Design review of the part built by this model. Coordinates are the model's own, in mm. A direction names the side the tool comes from. Coordinates: 2 decimals unless noted, no trailing zeros. Write each loop counter-clockwise with the first axis right and the second up, starting at its lowest first coordinate (ties: lowest second). Pieces come first, ordered by that corner, then holes.
Q1. Take a section at D-D, the plane z = 0. Write out the cut boundary in (x, y).
Q2. For pin 1 Ø5 at (x, z) = (14.5, -1.5) entering from -Y; pin 2 Ø3 at (y, z) = (4.5, 2) entering from +X; pin 3 Ø3 at (y, z) = (3, 0.5) entering from -X; pin 4 Ø1.5 at (x, z) = (-14, -3.5) entering from -Y, all flat-tipped, find the tip position at first contact; note any pin that passes through.
Q3. For L1, parallel to X at y = 0.45, z = -3.5; L2, parallel to Y at x = 13, z = -5; L3, parallel to X at y = -8, z = -3.5, list the stretches that pass through material, from the lowest coordinate up.
Q4. For faces 1 (the flat face through (-16, 0.5, 0.1)), 2 (the flat face through (-14, 1, 0)), 3 (the cylindrical face through (-10.53, 7.09, -1.08)), 4 (the flat face through (14, 0, 0)), 5 (the flat face through (-14, 0, 0)), list the 3-axis set-ups (+Z, -Z, +X, -X, +Y, -Y) from which the entire face can be reached by the end or side of a thin tool; tool diameter is ignored.
Q5. The part is to be moulded in two halves that separate along Z. For faces 6 (the flat face through (0, -7, -6)), 7 (the cylindrical face through (-12.946, 0.493, 4.172)), 8 (the cylindrical face through (-12.946, 0.493, -2.828)), 9 (the cylindrical face through (-7.87, 9.37, 1.15)), say which applies: released by +Z, released by -Z, zero draft, split by the parting line, or undercut.
Q6. Take a section at A-A, the plane x = 14. Write out the cut boundary in (y, z), plus the area to 3 significant figures.
Q7. Take a section at B-B, the plane z = -3.75. Write out the cut boundary in (x, y), plus the area to 3 significant figures.
Q8. Take a section at C-C, the plane x = -5.65. Write out the cut boundary in (y, z).
from build123d import *

# Parameters (mm, degrees)
EXTRUDE_1_DEPTH      = 6.6
EXTRUDE_1_DEPTH_BACK = 19.8
SKETCH_1_W           = 23
SKETCH_1_H           = 12
SKETCH_1_3_W         = 4.5
SKETCH_1_3_H         = 12
SKETCH_1_3_R         = 1.25
EXTRUDE_2_DEPTH      = 1
SKETCH_2_R           = 2.5
EXTRUDE_3_DEPTH      = 4.6
SKETCH_3_R           = 5
EXTRUDE_4_DEPTH      = 1


with BuildPart() as part:
    # Sketch 1 → Extrude 1 (new, two sides: drawn at the far end of the back side and taken through both)
    with BuildSketch(Plane(origin=(0, 0, 0), x_dir=(1, 0, 0), z_dir=(0, 1, 0)).offset(-EXTRUDE_1_DEPTH_BACK)):
        Rectangle(SKETCH_1_W, SKETCH_1_H)
    extrude(amount=EXTRUDE_1_DEPTH + EXTRUDE_1_DEPTH_BACK)

    # Sketch 1_3 → Extrude 2 (add)
    # profile 1 of 2: a face of its own
    with BuildSketch(Plane(origin=(0, 0, 0), x_dir=(1, 0, 0), z_dir=(0, 1, 0))):
        with Locations((13.75, 0)):
            Rectangle(SKETCH_1_3_W, SKETCH_1_3_H)
        with Locations(Location((14, -3.5, 0), (0, 0, 270))):
            Circle(SKETCH_1_3_R, mode=Mode.SUBTRACT)
        with Locations(Location((14, 3.5, 0), (0, 0, 270))):
            Circle(SKETCH_1_3_R, mode=Mode.SUBTRACT)
    # profile 2 of 2: a face of its own
    with BuildSketch(Plane(origin=(0, 0, 0), x_dir=(1, 0, 0), z_dir=(0, 1, 0))):
        with Locations((-13.75, 0)):
            Rectangle(SKETCH_1_3_W, SKETCH_1_3_H)
        with Locations(Location((-14, -3.5, 0), (0, 0, 270))):
            Circle(SKETCH_1_3_R, mode=Mode.SUBTRACT)
        with Locations(Location((-14, 3.5, 0), (0, 0, 270))):
            Circle(SKETCH_1_3_R, mode=Mode.SUBTRACT)
    extrude(amount=EXTRUDE_2_DEPTH)

    # Sketch 2 → Extrude 3 (add)
    with BuildSketch(Plane(origin=(0, 6.6, 0), x_dir=(1, 0, 0), z_dir=(0, 1, 0))):
        with Locations(Location((-5.65, 0, 0), (0, 0, 270))):
            Circle(SKETCH_2_R)
    extrude(amount=EXTRUDE_3_DEPTH)

    # Sketch 3 → Extrude 4 (add)
    with BuildSketch(Plane(origin=(0, 6.6, 0), x_dir=(1, 0, 0), z_dir=(0, 1, 0))):
        with Locations(Location((-5.65, 0, 0), (0, 0, 270))):
            Circle(SKETCH_3_R)
    extrude(amount=EXTRUDE_4_DEPTH)


solid = part.part
Responses:
1. outline: (-16, 0) - (-11.5, 0) - (-11.5, -19.8) - (11.5, -19.8) - (11.5, 0) - (16, 0) - (16, 1) - (11.5, 1) - (11.5, 6.6) - (-0.65, 6.6) - (-0.65, 7.6) - (-3.15, 7.6) - (-3.15, 11.2) - (-8.15, 11.2) - (-8.15, 7.6) - (-10.65, 7.6) - (-10.65, 6.6) - (-11.5, 6.6) - (-11.5, 1) - (-16, 1) - close
2. pin 1: stops at y = 0
2. pin 2: stops at x = 11.5
2. pin 3: stops at x = -11.5
2. pin 4: passes through
3. L1: x = -16 to -15.25, -12.75 to 12.75, 15.25 to 16
3. L2: y = 0 to 1
3. L3: x = -11.5 to 11.5
4. face 1: +Z, -Z, -X, +Y, -Y
4. face 2: +Z, -Z, -X, +Y
4. face 3: +Y
4. face 4: +Z, -Z, +X, -Y
4. face 5: +Z, -Z, -X, -Y
5. face 6: released by -Z
5. face 7: undercut
5. face 8: undercut
5. face 9: split by the parting line
6. outline: (0, -6) - (1, -6) - (1, -4.75) - (0, -4.75) - close; (0, -2.25) - (1, -2.25) - (1, 2.25) - (0, 2.25) - close; (0, 4.75) - (1, 4.75) - (1, 6) - (0, 6) - close
6. area: 7.00 mm2
7. outline: (-16, 0) - (-15.22, 0) - (-15.22, 1) - (-16, 1) - close; (-12.78, 0) - (-11.5, 0) - (-11.5, -19.8) - (11.5, -19.8) - (11.5, 0) - (12.78, 0) - (12.78, 1) - (11.5, 1) - (11.5, 6.6) - (-2.34, 6.6) - (-2.34, 7.6) - (-8.96, 7.6) - (-8.96, 6.6) - (-11.5, 6.6) - (-11.5, 1) - (-12.78, 1) - close; (15.22, 0) - (16, 0) - (16, 1) - (15.22, 1) - close
7. area: 618 mm2
8. outline: (-19.8, -6) - (6.6, -6) - (6.6, -5) - (7.6, -5) - (7.6, -2.5) - (11.2, -2.5) - (11.2, 2.5) - (7.6, 2.5) - (7.6, 5) - (6.6, 5) - (6.6, 6) - (-19.8, 6) - close
